The listing builds one solid part. Answer for the finished solid, in the listing's coordinates (mm). Face numbers are marked on the shaded views. A direction names the side the tool comes from. Give positions to 0.01 mm unless a question says otherwise; leave off trailing zeros. Loops run counter-clockwise (first coordinate to the right, second up) from the corner with the lowest first, then second, coordinate; pieces in that order, holes last. Notation, with made-up numbers: (72, 42.5) - (122, 42.5) arc R24 ccw to (122, 59.5) - close; hole circle Ø3 at (52.5, 67). An arc over 180 degrees is marked (long way). Answer as CSV lines item,"result". Start each with the question number.
1) Flat-ended cylindrical pins translate along their axes: pin 1 (1.5 mm diameter, centred on x = -1, y = 0, fed in from +Z); pin 2 (5 mm diameter, centred on y = 4, z = -7, fed in from +X); pin 3 (3 mm diameter, centred on x = 2.5, z = -20, fed in from -Y). Find the tip coordinate at first contact, or state that the pin passes through.
2) For the marked faces 1 and 2, determine the directions among +Z, -Z, +X, -X, +Y, -Y from which every point of the face is accessible in a straight line to the end or side of a thin tool.
3) For a pull along Y with two mould halves and no side action, classify the marked faces 3, 4, 5 and 6 as pulls with the +Y half, pulls with the -Y half, needs draft (parallel to the pull), parting line crosses it, or undercut.
4) A cutting plane is placed at B-B (z = -19.5). Determine the outline of the cut face in (x, y).
5) Find the intervals of material crossed by line 1 along Y through (x, z) = (0, -2) (3 decimals); line 2 along Z through (x, y) = (0.5, 5.25); line 3 along Z through (x, y) = (-3.25, -0.25), in increasing order.
6) A cutting plane is placed at A-A (z = -13). Determine the outline of the cut face in (x, y), and give its area (3 significant figures).
Autodesk Inventor part; units mm, degrees
ref_plane "MSC_PF1" through (0, 0, 0) normal (0, 1, 0) x (-1, 0, 0)
ref_plane "MSC_PT1" through (0, 0, -6.578) normal (0, 0, -1) x (-1, 0, 0)
ref_plane "YZ Plane" through (0, 0, 0) normal (1, 0, 0) x (0, 1, 0)
sketch "Sketch2" plane through (0, 0, 0) normal (0, 1, 0) x (-1, 0, 0)
  line L0 (0, -6.578) -> (0, -36.578)
  line L1 (0, -36.578) -> (3.375, -36.578)
  line L2 (4, -35.953) -> (4, -14.578)
  line L3 (4, -14.578) -> (3.55, -13.7986)
  line L4 (3.55, -13.7986) -> (3.55, -6.578)
  line L5 (3.55, -6.578) -> (0, -6.578)
  line L6 (3.375, -36.578) -> (4, -35.953)
  line L7 (4, -36.578) -> (4, -37.4619)
  line L8 (0, -43.6386) -> (0, -0.4012)
  dimension "Ds" = 7.1
  dimension "NND" = 8
  dimension "b" = 22
  dimension "d3" = 30
  dimension "d5" = 45
  dimension "PTC" = 1.25
  dimension "NLG" = 30
revolve "Revolution1" add sketch "Sketch2" angle 360 about axis through (0, 0, -6.578) along (0, 0, -1)
sketch "Sketch3" plane through (0, 0, -6.578) normal (0, 0, 1) x (1, 0, 0)
  circle A0 centre (0, 0) radius 3.55
  line L0 (0, 6.5) -> (3.7528, 6.5)
  line L1 (3.7528, 6.5) -> (7.5056, 0)
  line L2 (7.5056, 0) -> (0, 0)
  line L3 (0, 0) -> (0, 6.5)
  line L4 (0, 6.5) -> (-3.7528, 6.5)
  line L5 (-3.7528, 6.5) -> (-7.5056, 0)
  line L6 (0, -6.5) -> (3.7528, -6.5)
  line L7 (3.7528, -6.5) -> (7.5056, 0)
  line L8 (-3.7528, -6.5) -> (-7.5056, 0)
  line L9 (0, -6.5) -> (-3.7528, -6.5)
  dimension "d9" = 60
  dimension "ParS" = 13
  dimension "msp_d11" = 13
extrude "Extrusion1" add sketch "Sketch3" along normal blind 5.3
sketch "Sketch4" plane through (0, 0, 0) normal (0, 1, 0) x (-1, 0, 0)
  line L0 (-6.5, -1.278) -> (-7.5056, -1.278)
  line L1 (-7.5056, -1.278) -> (-7.5056, -1.8585)
  line L2 (-7.5056, -1.8585) -> (-6.5, -1.278)
  line L3 (0, -13.4454) -> (0, 34.6268)
  line L4 (0, 27.7593) -> (0, 27.1787)
  line L5 (-7.5056, -6.578) -> (-7.5056, -1.278)
  line L6 (-3.7528, -1.278) -> (-7.5056, -1.278)
  dimension "d14" = 30
  dimension "msp_d15" = 13
revolve "Revolution2" cut sketch "Sketch4" angle 360 about axis through (0, 0, 27.7593) along (0, 0, -1)
sketch "Sketch5" plane through (0, 0, -1.278) normal (0, 0, 1) x (1, 0, 0)
  arc A0 (5.6292, 3.25) -> (0, 6.5) centre (0, 0) ccw
  circle A1 centre (0, 0) radius 4.875
  dimension "d27" = 9.75
extrude "Extrusion2" cut sketch "Sketch5" against normal blind 1.06
thread "Thread1"
ref_plane "MSC_PF1" through (0, 0, 0) normal (0, 1, 0) x (-1, 0, 0)
ref_plane "MSC_PT1" through (0, 0, -6.578) normal (0, 0, -1) x (-1, 0, 0)
fillet "Fillet1" radius 0.4 1 edges at (3.55, 0, -6.578)
equation "\"msp_d11\" = ParS"
equation "\"msp_d15\" = ParS"
equation "\"d27\" = 0.75 * ParS"
equation "\"d28\" = 0.2 * ParK"
equation "\"d30\" = r"
equation "\"msp_d17\" = b"
equation "\"r\" = 0.4"
equation "\"THREADDIA\" = NND"
properties part number "ISO 4015 - M8 x 30" material "Stainless Steel, 440C"
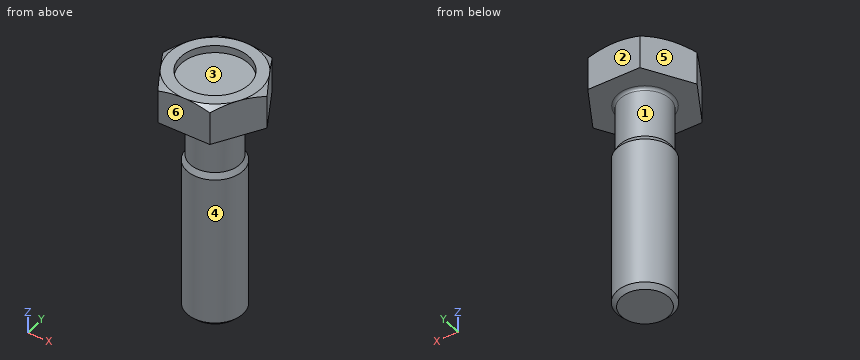
Ans:
1,pin 1,"z = -2.34"
1,pin 2,"x = 6.62"
1,pin 3,"y = -3.87"
2,face 1,"none"
2,face 2,"+Z, -Z, +X, -X, +Y"
3,face 3,"undercut"
3,face 4,"parting line crosses it"
3,face 5,"pulls with the +Y half"
3,face 6,"pulls with the -Y half"
4,outline,"circle Ø8 at (0, 0)"
5,line 1,"-6.5 to -4.875, 4.875 to 6.5"
5,line 2,"-6.58 to -1.28"
5,line 3,"-36.58 to -2.34"
6,outline,"circle Ø7.1 at (0, 0)"
6,area,"39.6 mm2"
